```python
from build123d import *

# Parameters (mm, degrees)
SKETCH1_R           = 10.16
BOSS_EXTRUDE1_DEPTH = 0.4
SKETCH2_R           = 5.8674
CUT_EXTRUDE1_DEPTH  = 15.373976485
CUT_EXTRUDE2_DEPTH  = 0.2


with BuildPart() as part:
    # Sketch1 → Boss-Extrude1 (new body)
    with BuildSketch(Plane(origin=(0, 0, 0), x_dir=(1, 0, 0), z_dir=(0, 1, 0))):
        with Locations(Location((0, 0, 0), (0, 0, 270))):
            Circle(SKETCH1_R)
    extrude(amount=BOSS_EXTRUDE1_DEPTH)

    # Sketch2 → Cut-Extrude1 (cut, through all)
    with BuildSketch(Plane(origin=(0, 0, 0), x_dir=(-1, 0, 0), z_dir=(0, -1, 0))):
        with Locations(Location((0, 0, 0), (0, 0, 90))):
            Circle(SKETCH2_R)
    extrude(amount=-CUT_EXTRUDE1_DEPTH, mode=Mode.SUBTRACT)

    # Sketch4 → Cut-Extrude2 (cut)
    # profile 1 of 3: a face of its own
    with BuildSketch(Plane(origin=(0, 0.4, 0), x_dir=(1, 0, 0), z_dir=(0, 1, 0))):
        with BuildLine():
            add(Edge.make_bspline(
                [(9.548097961, 1.097469618), (9.550055121, 1.073968459), (9.553888422, 1.027939027), (9.554390186, 0.959782463), (9.550385332, 0.894277853), (9.543161692, 0.830950704), (9.529924907, 0.770564877), (9.514466283, 0.712015933), (9.493128413, 0.656576452), (9.46859878, 0.603112304), (9.438240587, 0.552630443), (9.403712845, 0.504076224), (9.363797313, 0.45815636), (9.318530635, 0.414953146), (9.268531255, 0.373440711), (9.212574881, 0.33528609), (9.152201079, 0.298537745), (9.086625336, 0.264527216), (9.015771284, 0.233035098), (8.939390022, 0.204332005), (8.85742296, 0.178713648), (8.770070519, 0.155516755), (8.677361705, 0.135213545), (8.579160422, 0.117686573), (8.475476658, 0.102717037), (8.40435551, 0.095299195), (8.367946051, 0.091501736)],
                knots=[0, 0, 0, 0, 0.959744186, 1.879757445, 2.771360733, 3.630433483, 4.470974874, 5.285729423, 6.092861057, 6.885868194, 7.677321799, 8.486806591, 9.30863703, 10.149710703, 11.031725224, 11.950856355, 12.90393232, 13.90755666, 14.955572763, 16.058595042, 17.227175211, 18.449982035, 19.736657795, 21.08935819, 22.509938377, 24, 24, 24, 24], degree=3))
            add(Edge.make_bspline(
                [(8.367946051, 0.091501736), (8.333424141, 0.088400085), (8.265746233, 0.082319503), (8.165677998, 0.079231171), (8.06952646, 0.077278789), (7.977053794, 0.081155481), (7.88830334, 0.087048161), (7.803306671, 0.098811355), (7.721736112, 0.11170348), (7.644437516, 0.130414375), (7.570830347, 0.151553041), (7.501385565, 0.177166916), (7.435509874, 0.205414386), (7.374430468, 0.238456025), (7.316418733, 0.273272083), (7.263625883, 0.313436527), (7.214343769, 0.356439358), (7.169055169, 0.402772658), (7.128001276, 0.452365342), (7.092229736, 0.505851447), (7.060066365, 0.561822042), (7.033139082, 0.62118597), (7.010403647, 0.683257406), (6.992100676, 0.748449734), (6.979079533, 0.816930644), (6.973464566, 0.863715974), (6.970615322, 0.887456597)],
                knots=[0, 0, 0, 0, 1.373964495, 2.693565985, 3.968553968, 5.185962309, 6.362128109, 7.493465967, 8.586945452, 9.634820339, 10.644545933, 11.621736809, 12.567827687, 13.483617295, 14.373243629, 15.247464012, 16.109610849, 16.964804151, 17.813643683, 18.658252232, 19.51307309, 20.370435758, 21.2393278, 22.1319618, 23.052087694, 24, 24, 24, 24], degree=3))
            add(Edge.make_bspline(
                [(6.970615322, 0.887456597), (6.968008966, 0.924187003), (6.962939891, 0.995623618), (6.968278191, 1.100187869), (6.982752186, 1.198611099), (7.008071475, 1.290725833), (7.04420274, 1.376531671), (7.090804819, 1.455803983), (7.147686668, 1.528817336), (7.215087504, 1.595277348), (7.293061596, 1.655917856), (7.382222508, 1.709460065), (7.481878053, 1.757653835), (7.592113819, 1.79993908), (7.713743669, 1.835405319), (7.845672722, 1.865615588), (7.988759307, 1.889211353), (8.087867057, 1.899976367), (8.139191711, 1.905551215)],
                knots=[0, 0, 0, 0, 0.999181933, 1.943299396, 2.836688392, 3.696188225, 4.530240668, 5.35776012, 6.186181664, 7.036493394, 7.921805995, 8.862264049, 9.85532249, 10.92466266, 12.06451709, 13.293082439, 14.598176172, 16, 16, 16, 16], degree=3))
            add(Edge.make_bspline(
                [(8.139191711, 1.905551215), (8.192076162, 1.909791843), (8.294429148, 1.917999186), (8.443873987, 1.920688736), (8.584142548, 1.915477705), (8.715338175, 1.902057842), (8.837357513, 1.88004073), (8.950319838, 1.850206381), (9.053768445, 1.810845774), (9.148284982, 1.764097891), (9.233267264, 1.708869395), (9.308278218, 1.645097177), (9.373256878, 1.573236551), (9.429154226, 1.493984326), (9.473668524, 1.40587554), (9.508962331, 1.310266213), (9.535431633, 1.206847242), (9.543804449, 1.134545408), (9.548097961, 1.097469618)],
                knots=[0, 0, 0, 0, 1.381791394, 2.674330027, 3.891007168, 5.036428095, 6.106690612, 7.117972597, 8.075364145, 8.985087285, 9.859944246, 10.708764313, 11.542333244, 12.37753583, 13.227367402, 14.105765436, 15.028652003, 16, 16, 16, 16], degree=3))
        make_face()
        with BuildLine():
            add(Edge.make_bspline(
                [(8.261561502, 0.646575521), (8.294456414, 0.649821856), (8.358447364, 0.656137), (8.451849855, 0.666375212), (8.539943244, 0.678399643), (8.622970291, 0.689310262), (8.700369127, 0.702561563), (8.772745842, 0.714744092), (8.839767332, 0.728682456), (8.901986015, 0.742841894), (8.959241455, 0.758465051), (9.012361258, 0.774117371), (9.061070952, 0.791611955), (9.106204362, 0.808792317), (9.147102593, 0.82752915), (9.183769707, 0.847406728), (9.216251369, 0.868414663), (9.253841893, 0.896112176), (9.292161978, 0.93470985), (9.324279971, 0.987899004), (9.341430959, 1.046837895), (9.339946559, 1.087265986), (9.33918737, 1.107942708)],
                knots=[0, 0, 0, 0, 1.559939649, 3.034573339, 4.433834629, 5.755759396, 6.985974602, 8.139252337, 9.219098498, 10.216076828, 11.149973839, 12.019543174, 12.828554085, 13.591800542, 14.297942877, 14.949827997, 15.558345547, 16.121961591, 17.152098737, 18.100852136, 19.028691373, 20, 20, 20, 20], degree=3))
            add(Edge.make_bspline(
                [(9.33918737, 1.107942708), (9.337640701, 1.119206946), (9.334605741, 1.141310259), (9.325241811, 1.172734036), (9.31176771, 1.201590004), (9.293873227, 1.227812058), (9.271323703, 1.251644445), (9.244711652, 1.274008937), (9.212873286, 1.293547355), (9.176637524, 1.311985124), (9.135144771, 1.328439431), (9.087936038, 1.342704924), (9.03486756, 1.354683111), (8.975778101, 1.364445967), (8.910136784, 1.372235916), (8.83765802, 1.377138278), (8.757841853, 1.378355959), (8.671282468, 1.377765829), (8.578631856, 1.375199821), (8.480728235, 1.369181036), (8.377787239, 1.362348998), (8.307484328, 1.355956026), (8.271483377, 1.352682292)],
                knots=[0, 0, 0, 0, 0.573306212, 1.12497326, 1.647738541, 2.175091007, 2.719775143, 3.2992746, 3.924540973, 4.60063781, 5.349821626, 6.17422386, 7.087672211, 8.09400518, 9.19609116, 10.423188986, 11.759030231, 13.224456304, 14.792560164, 16.436793354, 18.175341204, 20, 20, 20, 20], degree=3))
            add(Edge.make_bspline(
                [(8.271483377, 1.352682292), (8.21872765, 1.347383023), (8.117512767, 1.337216074), (7.972444719, 1.319230054), (7.840842152, 1.298928139), (7.722599788, 1.277041996), (7.617710788, 1.253595709), (7.525847566, 1.228398034), (7.447076026, 1.201897522), (7.380933906, 1.17356744), (7.325919961, 1.144098193), (7.28035653, 1.113538037), (7.243905652, 1.081205208), (7.215355923, 1.047943532), (7.195791651, 1.012267519), (7.182777989, 0.975237705), (7.176443594, 0.935977323), (7.177754028, 0.909335291), (7.178423481, 0.895724826)],
                knots=[0, 0, 0, 0, 1.987774042, 3.813658246, 5.479624312, 6.979295976, 8.321212524, 9.507797241, 10.549079436, 11.434594746, 12.202068828, 12.886080949, 13.486172645, 14.024182533, 14.520633445, 15.002090577, 15.490203663, 16, 16, 16, 16], degree=3))
            add(Edge.make_bspline(
                [(7.178423481, 0.895724826), (7.18057015, 0.880150586), (7.184763265, 0.849729237), (7.201322999, 0.807002831), (7.225450517, 0.768795664), (7.257660898, 0.735091078), (7.298058684, 0.706441494), (7.346173767, 0.682368855), (7.401776004, 0.661890172), (7.465624388, 0.646320653), (7.537344011, 0.634570729), (7.61681871, 0.625748345), (7.704218452, 0.620988642), (7.799654696, 0.620157169), (7.90331396, 0.622569433), (8.015409368, 0.627671035), (8.13581459, 0.635163946), (8.218766894, 0.642691896), (8.261561502, 0.646575521)],
                knots=[0, 0, 0, 0, 0.622531695, 1.215998619, 1.802972471, 2.4067536, 3.054715399, 3.759494987, 4.537400922, 5.402670149, 6.364594255, 7.421637757, 8.576224243, 9.838461732, 11.210360544, 12.692839009, 14.293854979, 16, 16, 16, 16], degree=3))
        make_face(mode=Mode.SUBTRACT)
    # profile 2 of 3: a face of its own
    with BuildSketch(Plane(origin=(0, 0.4, 0), x_dir=(1, 0, 0), z_dir=(0, 1, 0))):
        Polygon((8.625595186, 2.745808752), (9.166888588, 2.901802676), (9.305794838, 2.420040523), (8.764501436, 2.264046599), align=None)
    # profile 3 of 3: a face of its own
    with BuildSketch(Plane(origin=(0, 0.4, 0), x_dir=(1, 0, 0), z_dir=(0, 1, 0))):
        with BuildLine():
            add(Edge.make_bspline(
                [(8.619317249, 3.839927612), (8.605158045, 3.855725986), (8.579584678, 3.884259905), (8.53958882, 3.918625978), (8.500604376, 3.943003738), (8.45722757, 3.951692461), (8.409998964, 3.948170804), (8.357468269, 3.932017987), (8.295899496, 3.907532011), (8.252095124, 3.887046328), (8.227954402, 3.875756605)],
                knots=[0, 0, 0, 0, 1.145744956, 2.069364517, 2.848247227, 3.600500716, 4.416765074, 5.385816981, 6.559315799, 8, 8, 8, 8], degree=3))
            Line((8.227954402, 3.875756605), (7.97604902, 3.75614289))
            Line((7.97604902, 3.75614289), (8.405996937, 2.851047404))
            Line((8.405996937, 2.851047404), (8.22354468, 2.764506605))
            Line((8.22354468, 2.764506605), (6.271691381, 3.093582126))
            Line((6.271691381, 3.093582126), (6.091443986, 3.473369452))
            Line((6.091443986, 3.473369452), (7.526257354, 4.154671536))
            Line((7.526257354, 4.154671536), (7.501452666, 4.207036987))
            add(Edge.make_bspline(
                [(7.501452666, 4.207036987), (7.495284595, 4.219752104), (7.483913694, 4.24319255), (7.467211949, 4.274824047), (7.45117189, 4.299250025), (7.432395351, 4.323142031), (7.404957274, 4.344998672), (7.371590737, 4.356451311), (7.340311976, 4.361880797), (7.310475748, 4.360944463), (7.275108034, 4.358439211), (7.249890175, 4.354257285), (7.236318118, 4.352006605)],
                knots=[0, 0, 0, 0, 1.244291285, 2.293863494, 3.146294454, 3.81324823, 4.96527056, 6.173175222, 6.877899736, 7.751404011, 8.789822906, 10, 10, 10, 10], degree=3))
            Line((7.236318118, 4.352006605), (7.15198218, 4.529497925))
            Line((7.15198218, 4.529497925), (7.534525583, 4.686043063))
            Line((7.534525583, 4.686043063), (7.739026451, 4.255543931))
            Line((7.739026451, 4.255543931), (7.990931833, 4.375157647))
            add(Edge.make_bspline(
                [(7.990931833, 4.375157647), (8.004889816, 4.382148034), (8.031410843, 4.395430199), (8.069069943, 4.414115601), (8.100867186, 4.433198132), (8.135895536, 4.454798796), (8.170657619, 4.48180517), (8.200545356, 4.517905625), (8.218913798, 4.556617267), (8.221958568, 4.600329456), (8.217615413, 4.648907387), (8.212529795, 4.683673908), (8.209764298, 4.702579522)],
                knots=[0, 0, 0, 0, 1.05478597, 2.004158271, 2.838732487, 3.558503911, 4.785687942, 5.791874313, 6.703150114, 7.627104706, 8.709648202, 10, 10, 10, 10], degree=3))
            Line((8.209764298, 4.702579522), (8.321109784, 4.755496188))
            Line((8.321109784, 4.755496188), (8.730662736, 3.892844279))
            Line((8.730662736, 3.892844279), (8.619317249, 3.839927612))
        make_face()
        with BuildLine():
            Line((8.037785131, 3.077596883), (7.763279923, 3.655270494))
            Line((7.763279923, 3.655270494), (7.376878013, 3.471715806))
            add(Edge.make_bspline(
                [(7.376878013, 3.471715806), (7.293366138, 3.433055727), (7.122021893, 3.353735487), (6.947231905, 3.282323746), (6.857633222, 3.245717543)],
                knots=[0, 0, 0, 0, 0.974784713, 2, 2, 2, 2], degree=3))
            Line((6.857633222, 3.245717543), (6.865350236, 3.229181084))
            Line((6.865350236, 3.229181084), (8.009121937, 3.063816501))
            Line((8.009121937, 3.063816501), (8.037785131, 3.077596883))
        make_face(mode=Mode.SUBTRACT)
    extrude(amount=-CUT_EXTRUDE2_DEPTH, mode=Mode.SUBTRACT)


solid = part.part
```
Can you work these out from the model? Positions are in its coordinate system, mm. Give positions to 0.01 mm unless a question says otherwise; leave off trailing zeros. Loops run counter-clockwise (first coordinate to the right, second up) from the corner with the lowest first, then second, coordinate; pieces in that order, holes last. Notation, with made-up numbers: M 40.25,-14 L 86.25,-14 A13 cw 86.25,8 Z; hole C 27.25,38.5 d11. An arc over 180 degrees is marked long. Answer in a Markdown table with one row per item.
1. Suppose I cut it at B-B on y = 0.3. Count the separate pieces of the cut face and the enclosed holes in it, plus the area to 3 significant figures.
Taken from the geometry:
| item | result |
|---|---|
| separate pieces | 3 |
| enclosed holes | 4 |
| area | 211 mm² |
2. If I drill on line 1 along X through (y, z) = (0.3, 0); line 2 along Z through (x, y) = (-0.25, 0.05); line 3 along X through (y, z) = (0.25, -4.5), over which ranges is the centre line in solid material (lowest first)?
Taken from the geometry:
| item | result |
|---|---|
| line 1 | x = -10.16 to -5.87, 5.87 to 10.16 |
| line 2 | z = -10.16 to -5.86, 5.86 to 10.16 |
| line 3 | x = -9.11 to -3.77, 3.77 to 7.17, 7.62 to 8.19, 8.44 to 9.11 |
3. For pin 1 Ø10.5 at (x, z) = (0, 0) entering from +Y, with a flat end and sliding along its axis, tell me the tip position at first contact or that it passes through.
Taken from the geometry:
| item | result |
|---|---|
| pin 1 | passes through |
4. Suppose I cut it at A-A on x = 0. Write out the boundary of the cut face in (y, z).
Taken from the geometry:
| item | result |
|---|---|
| outline | M 0,-10.16 L 0.4,-10.16 L 0.4,-5.87 L 0,-5.87 Z; M 0,5.87 L 0.4,5.87 L 0.4,10.16 L 0,10.16 Z |
5. Suppose I cut it at D-D on z = 8.5. Write out the boundary of the cut face in (x, y).
Taken from the geometry:
| item | result |
|---|---|
| outline | M -5.57,0 L 5.57,0 L 5.57,0.4 L -5.57,0.4 Z |
6. Thinking about a two-plate mould opening in X: for faces 1 (the flat face through (7.4, 0.2, -3.8)), 2 (the cylindrical face through (10.074, 0.197, -1.323)), 3 (the flat face through (-4.4, 0.4, 4.4)), which applies, released by +X, released by -X, zero draft, split by the parting line, or undercut?
Taken from the geometry:
| item | result |
|---|---|
| face 1 | undercut |
| face 2 | split by the parting line |
| face 3 | zero draft |
7. Suppose I cut it at C-C on z = 0.5. Write out the boundary of the cut face in (x, y), plus the area to 3 significant figures.
Taken from the geometry:
| item | result |
|---|---|
| outline | M -10.15,0 L -5.85,0 L -5.85,0.4 L -10.15,0.4 Z; M 5.85,0 L 10.15,0 L 10.15,0.4 L 5.85,0.4 Z |
| area | 3.44 mm² |
